from build123d import *

# Parameters (mm, degrees)
M4_CLEARANCE_HOLE1_D     = 4.5
M4_CLEARANCE_HOLE1_DEPTH = 10
M4_CLEARANCE_HOLE1_TIP   = 1.351936393
FILLET1_R                = 0.2
CHAMFER1_SIZE            = 0.5


with BuildPart() as part:
    # Sketch1 → Revolve1 (revolve)
    with BuildSketch(Plane.XY, mode=Mode.PRIVATE) as revolve1_sk:
        Polygon((9, 0), (31, 0), (31, 5), (16, 5), (16, 46.85), (11, 46.85), (11, 8.85), (9, 8.85), align=None)
    revolve(revolve1_sk.sketch.rotate(Axis((0, 9.488188976, 0), (0, -1, 0)), 90), axis=Axis((0, 9.488188976, 0), (0, -1, 0)))

    # M4 Clearance Hole1
    with Locations(Plane(origin=(0, 5, 0), x_dir=(1, 0, 0), z_dir=(0, 1, 0))):
        with Locations((23.5, 0), (0, 23.5), (0, -23.5), (-23.5, 0)):
            Hole(M4_CLEARANCE_HOLE1_D / 2, depth=M4_CLEARANCE_HOLE1_DEPTH)
            with Locations((0, 0, -(M4_CLEARANCE_HOLE1_DEPTH + M4_CLEARANCE_HOLE1_TIP / 2))):  # 118° drill point
                Cone(0, M4_CLEARANCE_HOLE1_D / 2, M4_CLEARANCE_HOLE1_TIP, mode=Mode.SUBTRACT)

    # Sketch5 → Groove for BS 3673 P4 - B022M, Internal Circlip1 (revolve, cut)
    with BuildSketch(Plane(origin=(0, 9.488188976, 0), x_dir=(0, 0, 1), z_dir=(-1, 0, 0))):
        with BuildLine():
            Line((11.39, 5.361811024), (9.9, 5.361811024))
            Line((9.9, 5.361811024), (9.9, 6.461811024))
            Line((9.9, 6.461811024), (11.39, 6.461811024))
            ThreePointArc((11.39, 6.461811024), (11.467781746, 6.42959277), (11.5, 6.351811024))
            Line((11.5, 6.351811024), (11.5, 5.471811024))
            ThreePointArc((11.5, 5.471811024), (11.467781746, 5.394029278), (11.39, 5.361811024))
        make_face()
    revolve(axis=Axis((0, -40.511811024, 0), (0, 1, 0)), mode=Mode.SUBTRACT)

    # Fillet1
    fillet1_edges = [part.edges().sort_by_distance(p)[0] for p in [
        (0, 8.85, -11),
        (0, 5, -16),
    ]]
    fillet(fillet1_edges, radius=FILLET1_R)

    # Chamfer1
    chamfer1_edges = [part.edges().sort_by_distance(p)[0] for p in [
        (0, 0, -9),
        (0, 8.85, -9),
        (0, 46.85, -11),
        (0, 46.85, -16),
        (0, 5, -31),
        (0, 0, -31),
    ]]
    chamfer(chamfer1_edges, length=CHAMFER1_SIZE)


solid = part.part
CAD build for the part. Positions are in the model's coordinates, mm. A direction names the side the tool comes from. Round coordinates to 2 decimals unless told otherwise and drop trailing zeros. Loops run counter-clockwise (first coordinate to the right, second up) from the corner with the lowest first, then second, coordinate; pieces in that order, holes last.
(1) Which spindle directions (+Z, -Z, +X, -X, +Y, -Y) get a long thin tool onto all of the face, cutting with end or side? Do faces 1 (the cylindrical face through (-6.083, 4.37, -6.633)), 2 (the flat face through (13, 5, 13)). Say none if no direction does.
(2) Cut at B-B (x = 1). State how many separate pieces and enclosed holes the cut face has, plus the area to 3 significant figures.
(3) Drop flat-ended pins along their axis: pin 1 (5 mm diameter, centred on x = -1.5, y = 32, fed in from -Z); pin 2 (5 mm diameter, centred on x = 0, z = 23.5, fed in from +Y); pin 3 (12 mm diameter, centred on x = 9.5, y = 28.5, fed in from -Z); pin 4 (18 mm diameter, centred on x = 1.5, z = 4.5, fed in from -Y). Give the stop position or say it passes through.
(4) Two-plate mould, pull along Y, no slides. Class faces 3 (the cylindrical face through (-30.736, 2.528, -4.036)), 4 (the cylindrical face through (11.4, 15.4, -1.5)), 5 (the flat face through (10, 8.85, 0)), 6 (the flat face through (-7, 0, 7)): +Y half, -Y half, draft (parallel to the pull), parting line (faces both ways), or undercut.
(5) Cut at A-A (y = 18). Give the cut face in (x, z).
(6) Wall check: line 1 along X through (y, z) = (15.2, 0); line 2 along X through (y, z) = (26, 0); line 3 along Y through (x, z) = (22.5, -15). Give the ranges that are in metal, low to high.
Findings below:
1. face 1: +Y, -Y
1. face 2: +Y
2. separate pieces: 4
2. enclosed holes: 0
2. area: 613 mm2
3. pin 1: stops at z = -16
3. pin 2: stops at y = 5
3. pin 3: stops at z = -15.61
3. pin 4: stops at y = 0
4. face 3: draft
4. face 4: undercut
4. face 5: +Y half
4. face 6: -Y half
5. outline: circle Ø32 at (0, 0); hole circle Ø22 at (0, 0)
6. line 1: x = -16 to -11.5, 11.5 to 16
6. line 2: x = -16 to -11, 11 to 16
6. line 3: y = 0 to 5
